Source: CAD feature listing. Evaluate the final solid. Frame: model axes, mm. Face numbers are marked on the shaded views. Give positions to 0.01 mm unless a question says otherwise; leave off trailing zeros. Write each loop counter-clockwise with the first axis right and the second up, starting at its lowest first coordinate (ties: lowest second). Pieces come first, ordered by that corner, then holes. Notation, with made-up numbers: (4, -38.5) -> (41, -38.5) arc R26 ccw to (41, -13.5) -> close; hole circle Ø11 at (-2.75, -4). An arc over 180 degrees is marked (long way). Write item = value, one per line.
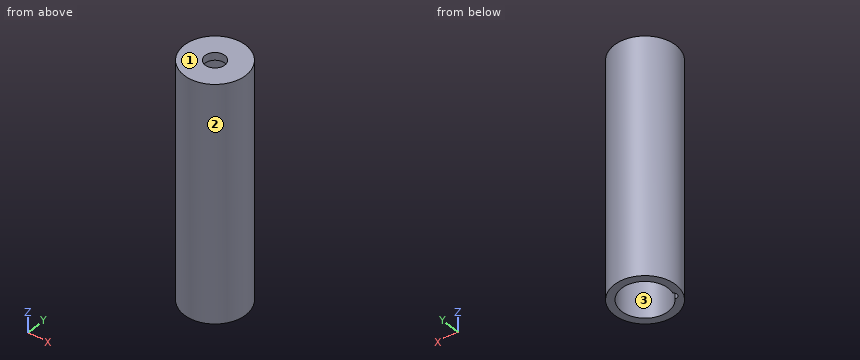
from build123d import *

# Parameters (mm, degrees)
F0_R     = 12.1
F0_R_2   = 3.875
F1_DEPTH = 3
F2_R     = 12.1
F3_DEPTH = 90


with BuildPart() as f1:
    # F0 (on Top) → F1 (new body)
    with BuildSketch(Plane.XY):
        Circle(F0_R)
        Circle(F0_R_2, mode=Mode.SUBTRACT)
    extrude(amount=F1_DEPTH)

    # F2 (on face) → F3 (join)
    with BuildSketch(Plane(origin=(0, 0, 0), x_dir=(1, 0, 0), z_dir=(0, 0, -1))):
        Circle(F2_R)
        with BuildLine():
            ThreePointArc((-8.819044, 2.620012), (-9.298069, 4.493539), (-7.532436, 5.282274))
            ThreePointArc((-7.532436, 5.282274), (8.283395, -4.00317), (-8.819044, 2.620012))
        make_face(mode=Mode.SUBTRACT)
    extrude(amount=F3_DEPTH)


solid = f1.part
1) Contact query for flat-ended pins moving along their axis: pin 1 (8 mm diameter, centred on x = -8.5, z = -40.5, fed in from +Y); pin 2 (5 mm diameter, centred on x = 0, y = 1, fed in from -Z); pin 3 (1 mm diameter, centred on y = 4, z = -26, fed in from +X); pin 4 (12.5 mm diameter, centred on x = 0, y = 0, fed in from -Z). Output: stop coordinate, or through.
Computed:
pin_1 = 11.23
pin_2 = through
pin_3 = 11.58
pin_4 = 0
2) Material intervals for L1, parallel to X at y = 0, z = -33; L2, parallel to Y at x = 6, z = -16.5, sorted ascending.
Computed:
L1 = -12.1 to -9.2, 9.2 to 12.1
L2 = -10.51 to -6.97, 6.97 to 10.51
3) Cut plane C-C (z = -78). Return the cut outline in (x, y), then the cut area to 3 significant figures.
Computed:
outline = circle Ø24.2 at (0, 0); hole (-8.82, -2.62) arc R1.5 ccw to (-7.53, -5.28) arc R9.2 ccw (long way) to start
area = 192 mm²
4) Cut plane B-B (x = 0). Return the cut outline in (y, z) (3 decimals).
Computed:
outline = (-12.1, -90) -> (-9.2, -90) -> (-9.2, 0) -> (-3.875, 0) -> (-3.875, 3) -> (-12.1, 3) -> close; (3.875, 0) -> (9.2, 0) -> (9.2, -90) -> (12.1, -90) -> (12.1, 3) -> (3.875, 3) -> close
5) Cut plane A-A (y = -1). Return the cut outline in (x, z), then the cut area to 3 significant figures.
Computed:
outline = (-12.06, -90) -> (-9.15, -90) -> (-9.15, 0) -> (-3.74, 0) -> (-3.74, 3) -> (-12.06, 3) -> close; (3.74, 0) -> (9.15, 0) -> (9.15, -90) -> (12.06, -90) -> (12.06, 3) -> (3.74, 3) -> close
area = 574 mm²
6) Draft query along X for the marked faces 1, 2 and 3. Return one class per face: pulls with the +X half, pulls with the -X half, needs draft (parallel to the pull), parting line crosses it, or undercut.
Computed:
face_1 = needs draft
face_2 = parting line crosses it
face_3 = undercut
7) Cut plane D-D (x = -5). Return the cut outline in (y, z).
Computed:
outline = (-11.02, -90) -> (-7.72, -90) -> (-7.72, 0) -> (7.72, 0) -> (7.72, -90) -> (11.02, -90) -> (11.02, 3) -> (-11.02, 3) -> close
